from build123d import *

# Parameters (mm, degrees)
BOSS_EXTRUDE1_DEPTH = 15


with BuildPart() as part:
    # Sketch1 → Boss-Extrude1 (new body)
    with BuildSketch(Plane.XY):
        with BuildLine():
            Line((-4.967004399, 8.835776472), (-71.884952029, -35.707198588))
            Line((-71.884952029, -35.707198588), (-86.833591926, -69.261290707))
            ThreePointArc((-86.833591926, -69.261290707), (-74.078855086, -82.121498504), (-61.218647289, -69.366761664))
            Line((-61.218647289, -69.366761664), (-54.340359202, -48.936608433))
            Line((-54.340359202, -48.936608433), (6.077760006, -5.382226646))
            Line((6.077760006, -5.382226646), (9.40798921, 2.245366823))
            Line((9.40798921, 2.245366823), (24.377091509, 13.963829782))
            Line((24.377091509, 13.963829782), (19.091883092, 19.091883092))
            Line((19.091883092, 19.091883092), (3.844956844, 8.835776472))
            Line((3.844956844, 8.835776472), (-4.967004399, 8.835776472))
        make_face()
    extrude(amount=-BOSS_EXTRUDE1_DEPTH)


solid = part.part
Verification items for the finished model (mm, model axes). A direction names the side the tool comes from. Round coordinates to 2 decimals unless told otherwise and drop trailing zeros. Loops run counter-clockwise (first coordinate to the right, second up) from the corner with the lowest first, then second, coordinate; pieces in that order, holes last. Notation, with made-up numbers: (27.5, 87) - (51.5, 87) arc R20 cw to (51.5, 117) - close; hole circle Ø1 at (-19.5, 23.5). An arc over 180 degrees is marked (long way). Answer in a Markdown table with one row per item. Add a question column.
Q1. Gauge pin test, flat ends, axial feed: pin 1 (5 mm diameter, centred on x = -28, z = -4.5, fed in from +Y); pin 2 (8 mm diameter, centred on x = -63, z = -5.5, fed in from +Y); pin 3 (7 mm diameter, centred on x = 0, z = -9, fed in from +Y). Record the tip position at first contact, or that the pin passes through.
Q2. Section check A-A on z = -7.25. Enter the section's corners in (x, y), plus the area to 3 significant figures.
Q3. Tool access check on faces 1 (the face through (0, 8.836, -7)), 2 (the face through (-44, -31, -15)). Record the directions out of +Z, -Z, +X, -X, +Y, -Y that give a thin tool (end or side, any length) a straight path to the whole face; none if there is none.
Q4. Section check B-B on y = 5.5. Enter the section's corners in (x, z), plus the area to 3 significant figures.
Q5. Material ranges on line 1 (X direction, y = -69.5, z = -3.25); line 2 (X direction, y = -3.5, z = -11); line 3 (Y direction, x = 1, z = -7), recorded low to high.
Q6. Section check C-C on x = -65. Enter the section's corners in (y, z).
Found:
| question | item | result |
|---|---|---|
| 1 | pin 1 | stops at y = -4.83 |
| 1 | pin 2 | stops at y = -27.13 |
| 1 | pin 3 | stops at y = 8.84 |
| 2 | outline | (-86.83, -69.26) arc R12.81 ccw to (-61.22, -69.37) - (-54.34, -48.94) - (6.08, -5.38) - (9.41, 2.25) - (24.38, 13.96) - (19.09, 19.09) - (3.84, 8.84) - (-4.97, 8.84) - (-71.88, -35.71) - close |
| 2 | area | 2,660 mm² |
| 3 | face 1 | +Z, -Z, -X, +Y |
| 3 | face 2 | -Z, +X, -X, +Y, -Y |
| 4 | outline | (-9.98, -15) - (13.57, -15) - (13.57, 0) - (-9.98, 0) - close |
| 4 | area | 353 mm² |
| 5 | line 1 | x = -86.83 to -61.22 |
| 5 | line 2 | x = -23.5 to 6.9 |
| 5 | line 3 | y = -9.04 to 8.84 |
| 6 | outline | (-78.4, -15) - (-31.12, -15) - (-31.12, 0) - (-78.4, 0) - close |
